Work out the finished part from the listing and answer in its coordinate system (mm). Face numbers are marked on the shaded views. A direction names the side the tool comes from. Coordinates: 2 decimals unless noted, no trailing zeros. Order: outer loops, then holes, each group sorted by start corner. A loop starts at its lowest first (then second) coordinate and runs counter-clockwise, first axis right, second up. Notation, with made-up numbers: M 25,-36 L 71,-36 A24 cw 71,-20 Z; hole C -20,56 d10. An arc over 180 degrees is marked long. Use a Markdown table: item, result.
from build123d import *

# Parameters (mm, degrees)
BOSS_EXTRUDE1_DEPTH      = 0.25
BOSS_EXTRUDE1_DEPTH_BACK = 14
SKETCH2_R                = 1.5
CUT_EXTRUDE1_DEPTH       = 14
SKETCH3_W                = 3.8
SKETCH3_H                = 25
BOSS_EXTRUDE2_DEPTH      = 10
CUT_EXTRUDE2_DEPTH       = 55.467329657
CUT_EXTRUDE2_DEPTH_BACK  = 55.467329657
SKETCH4_R                = 1.5
SKETCH4_W                = 7
SKETCH4_H                = 8.5
FILLET1_R                = 4
FILLET2_R                = 2.5
SKETCH5_W                = 8
SKETCH5_H                = 25
CUT_EXTRUDE3_DEPTH       = 1.8
FILLET3_R                = 3
FILLET4_R                = 3


with BuildPart() as part:
    # Sketch1 → Boss-Extrude1 (new, two sides: drawn at the far end of the back side and taken through both)
    with BuildSketch(Plane.XY.offset(-BOSS_EXTRUDE1_DEPTH_BACK)):
        Polygon((-23.42202285, 43.125), (-23.42202285, 45.25), (-21.850576241, 45.25), (-19.62202285, 43.021446609), (-19.62202285, 36.978553391), (-21.850576241, 34.75), (-23.42202285, 34.75), align=None)
    extrude(amount=BOSS_EXTRUDE1_DEPTH + BOSS_EXTRUDE1_DEPTH_BACK)

    # Sketch2 → Cut-Extrude1 (cut)
    with BuildSketch(Plane.ZY.offset(23.42202285)):
        with Locations((-5.863626805, 40)):
            Circle(SKETCH2_R)
    extrude(amount=-CUT_EXTRUDE1_DEPTH, mode=Mode.SUBTRACT)

    # Sketch3 → Boss-Extrude2 (add)
    with BuildSketch(Plane.XY.offset(0.25)):
        with Locations((-21.52202285, 40)):
            Rectangle(SKETCH3_W, SKETCH3_H)
    extrude(amount=BOSS_EXTRUDE2_DEPTH)

    # Sketch4 → Cut-Extrude2 (cut, two sides: drawn at the far end of the back side and taken through both)
    with BuildSketch(Plane.ZY.offset(23.42202285).offset(-CUT_EXTRUDE2_DEPTH_BACK)):
        with Locations((6.25, 47.75)):
            Circle(SKETCH4_R)
        with Locations((6.25, 32.25)):
            Circle(SKETCH4_R)
        with Locations((6.75, 40)):
            Rectangle(SKETCH4_W, SKETCH4_H)
    extrude(amount=CUT_EXTRUDE2_DEPTH + CUT_EXTRUDE2_DEPTH_BACK, mode=Mode.SUBTRACT)

    # Fillet1
    fillet1_edges = [part.edges().sort_by_distance(p)[0] for p in [
        (-21.52202285, 27.5, 0.25),
        (-21.52202285, 52.5, 0.25),
        (-21.52202285, 27.5, 10.25),
        (-21.52202285, 52.5, 10.25),
    ]]
    fillet(fillet1_edges, radius=FILLET1_R)

    # Fillet2
    fillet2_edges = [part.edges().sort_by_distance(p)[0] for p in [
        (-21.52202285, 35.75, 3.25),
        (-21.52202285, 44.25, 3.25),
    ]]
    fillet(fillet2_edges, radius=FILLET2_R)

    # Sketch5 → Cut-Extrude3 (cut)
    with BuildSketch(Plane(origin=(-19.62202285, 0, 0), x_dir=(0, 0, -1), z_dir=(1, 0, 0))):
        with Locations((-6.25, 40)):
            Rectangle(SKETCH5_W, SKETCH5_H)
    extrude(amount=-CUT_EXTRUDE3_DEPTH, mode=Mode.SUBTRACT)

    # Fillet3
    # the kernel refuses this fillet: 3 mm, written as the material it takes off along each edge
    with BuildSketch(Plane(origin=(-19.62202285, 58.837965158, 2.25), x_dir=(-1, 0, 0), z_dir=(0, -1, 0))) as fillet3_piece_1:
        with BuildLine():
            CenterArc((3, 2.749545417), FILLET3_R, 180, 66.421821522)
            Line((0, 2.749545417), (-0.06, 2.749545417))
            Line((-0.06, 2.749545417), (-0.06, 0))
            Line((-0.06, 0), (0, -0.06))
            ThreePointArc((0, -0.06), (0.9, -0.06), (1.776, -0.054990908))
            Line((1.776, -0.054990908), (1.8, 0))
        make_face()
    extrude(amount=37.675930315, mode=Mode.SUBTRACT)

    # Fillet4
    fillet4_edges = [part.edges().sort_by_distance(p)[0] for p in [
        (-21.42202285, 40, 2.25),
    ]]
    fillet(fillet4_edges, radius=FILLET4_R)


solid = part.part
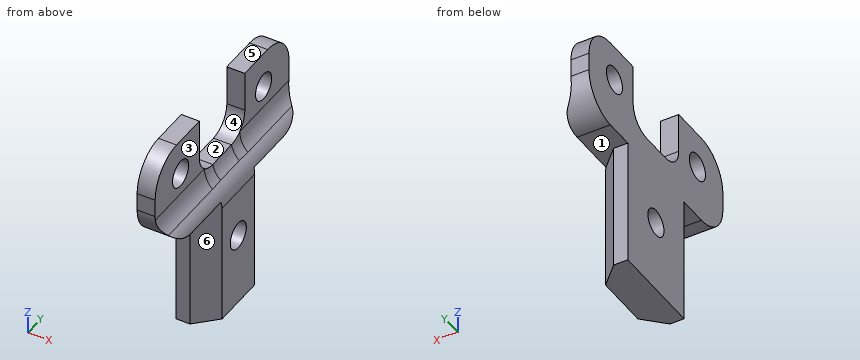
(1) Determine the mould class of the marked faces 4, 5 and 6 for opening direction Y: pulls with the +Y half, pulls with the -Y half, needs draft (parallel to the pull), parting line crosses it, or undercut.
Conclusion:
| item | result |
|---|---|
| face 4 | undercut |
| face 5 | needs draft |
| face 6 | pulls with the -Y half |
(2) A cutting plane is placed at B-B (z = -9.5). Determine the outline of the cut face in (x, y).
Conclusion:
| item | result |
|---|---|
| outline | M -23.42,34.75 L -21.85,34.75 L -19.62,36.98 L -19.62,43.02 L -21.85,45.25 L -23.42,45.25 Z |
(3) Which of the six approach directions +Z, -Z, +X, -X, +Y, -Y give full straight-line access (tool end or side, diameter ignored) to the marked faces 1, 2 and 3?
Conclusion:
| item | result |
|---|---|
| face 1 | -Z, +X, +Y |
| face 2 | +Z, +X, -X |
| face 3 | +Z, +X, +Y, -Y |
(4) Given P1, Ø5, axis at y = 31.5, z = 6.5, coming from the +X side; P2, Ø1.8, axis at y = 40, z = -5.86, coming from the +X side; P3, Ø0.6, axis at x = -22, z = 7.5, coming from the +Y side; P4, Ø1, axis at x = -22.5, y = 40, coming from the +Z side, each flat-ended and moving along its own axis, determine where each tip first touches the part or whether it passes through.
Conclusion:
| item | result |
|---|---|
| P1 | x = -21.42 |
| P2 | through |
| P3 | y = 52.39 |
| P4 | z = 3.25 |
(5) A cutting plane is placed at A-A (y = 32.25). Determine the outline of the cut face in (x, z).
Conclusion:
| item | result |
|---|---|
| outline | M -23.42,0.25 L -19.72,0.25 A3 ccw -20.52,1.64 A3 cw -21.42,3.79 L -21.42,4.75 L -23.42,4.75 Z; M -23.42,7.75 L -21.42,7.75 L -21.42,10.25 L -23.42,10.25 Z |
(6) Straight lines are drawn through the part: L1, parallel to Y at x = -21.95, z = -10.5; L2, parallel to Z at x = -22.25, y = 32.25; L3, parallel to Z at x = -22.65, y = 46.5. For each, find the intervals that lie inside material, in ascending order.
Conclusion:
| item | result |
|---|---|
| L1 | 34.75 to 45.25 |
| L2 | 0.25 to 4.75, 7.75 to 10.25 |
| L3 | 0.25 to 5.42, 7.08 to 10.25 |
